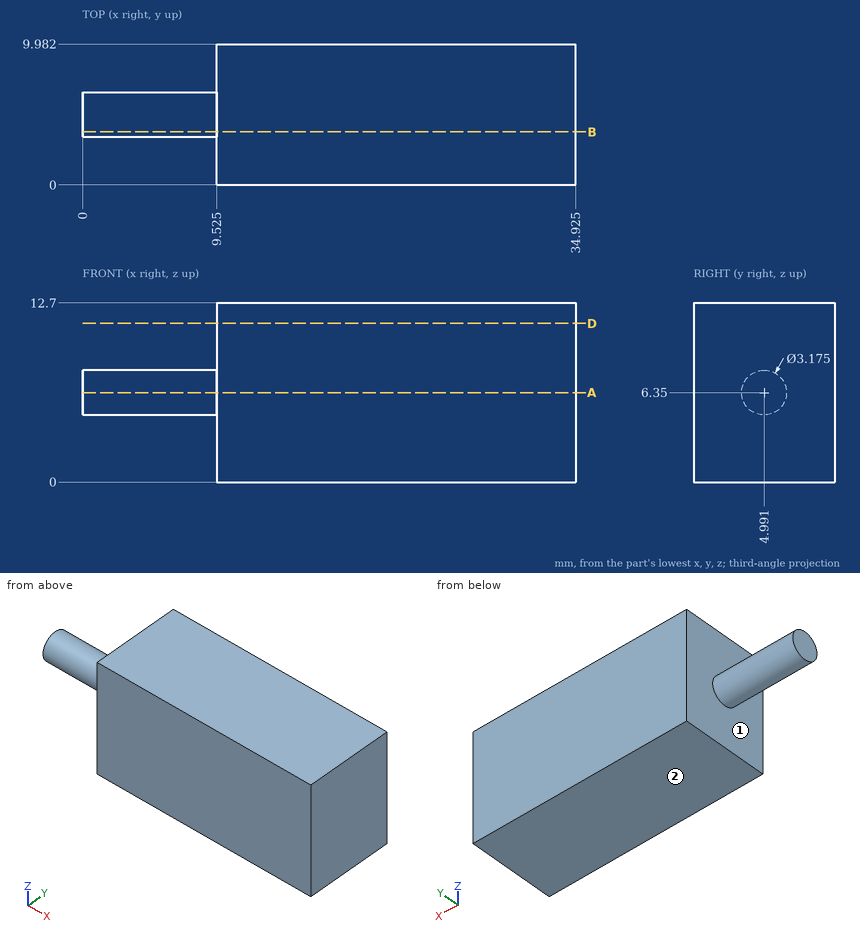
Geometry check sheet. Reference: drawing and pictorial views, mm from the part's lowest x, y, z. A direction names the side the tool comes from. Coordinates: 2 decimals unless noted, no trailing zeros. Write each loop counter-clockwise with the first axis right and the second up, starting at its lowest first coordinate (ties: lowest second). Pieces come first, ordered by that corner, then holes. Notation, with made-up numbers: (-9.5, -16) - (23.5, -16) arc R11 cw to (23.5, 2) - close; hole circle Ø2 at (24.25, -12.75). An arc over 180 degrees is marked (long way). Write item = value, one per line.
Q1. Cross-section at D-D (z = 11.25). Enter the section's corners in (x, y) (1 decimal), plus the area to 3 significant figures.
Answer:
outline = (9.5, 0) - (34.9, 0) - (34.9, 10) - (9.5, 10) - close
area = 254 mm²
Q2. Access from +Z, -Z, +X, -X, +Y, -Y to the whole of each face (thin tool, end or side, straight path). Record for the marked faces 1 and 2.
Answer:
face_1 = -X
face_2 = -Z, +X, -X, +Y, -Y
Q3. Cross-section at B-B (y = 3.75). Enter the section's corners in (x, z) (1 decimal).
Answer:
outline = (0, 5.4) - (9.5, 5.4) - (9.5, 0) - (34.9, 0) - (34.9, 12.7) - (9.5, 12.7) - (9.5, 7.3) - (0, 7.3) - close
Q4. Cross-section at A-A (z = 6.35). Enter the section's corners in (x, y) (1 decimal), plus the area to 3 significant figures.
Answer:
outline = (0, 3.4) - (9.5, 3.4) - (9.5, 0) - (34.9, 0) - (34.9, 10) - (9.5, 10) - (9.5, 6.6) - (0, 6.6) - close
area = 284 mm²
Q5. Go/stop test with a flat-tipped pin: pin 1 Ø2 at (y, z) = (4, 3.5) entering from -X (3 decimals). Record where the tip stops, or that it passes through.
Answer:
pin_1 = 9.525
Q6. Material ranges on L1, parallel to X at y = 0.5, z = 5.25 (3 decimals); L2, parallel to Y at x = 5.5, z = 7, recorded low to high. Write a range as from..to.
Answer:
L1 = 9.525..34.925
L2 = 3.54..6.44
